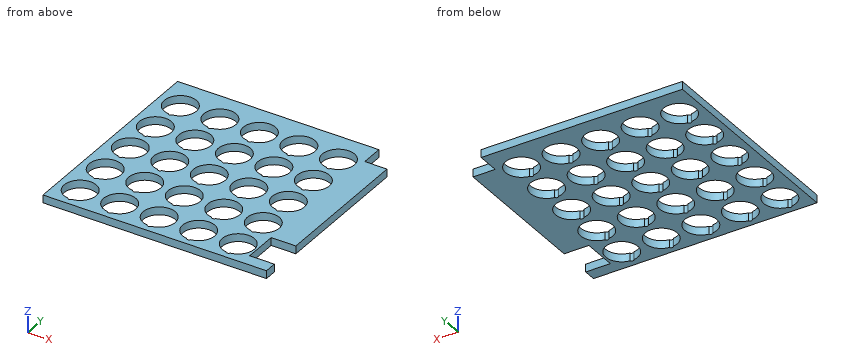
```python
from build123d import *

# Parameters (mm, degrees)
SKETCH2_W           = 180.975
SKETCH2_H           = 161.925
BOSS_EXTRUDE1_DEPTH = 6.35
SKETCH6_W           = 180.975
SKETCH6_H           = 10
BOSS_EXTRUDE2_DEPTH = 6.35
SKETCH3_R           = 13
CUT_EXTRUDE1_DEPTH  = 243.923812645
SKETCH4_R           = 1.75
CUT_EXTRUDE9_DEPTH  = 243.923812645
SKETCH7_W           = 20
SKETCH7_H           = 27.5
SKETCH7_W_2         = 18
SKETCH7_H_2         = 18
CUT_EXTRUDE10_DEPTH = 243.923812645


with BuildPart() as part:
    # Sketch2 → Boss-Extrude1 (new body)
    with BuildSketch(Plane.XY):
        with Locations((90.4875, 80.9625)):
            Rectangle(SKETCH2_W, SKETCH2_H)
    extrude(amount=BOSS_EXTRUDE1_DEPTH)

    # Sketch6 → Boss-Extrude2 (add)
    with BuildSketch(Plane.XY.offset(6.35)):
        with Locations((90.4875, -5)):
            Rectangle(SKETCH6_W, SKETCH6_H)
    extrude(amount=-BOSS_EXTRUDE2_DEPTH)

    # Sketch3 → Cut-Extrude1 (cut, through all)
    with BuildSketch(Plane.XY.offset(6.35)):
        with Locations((18.25, 8.675)):
            Circle(SKETCH3_R)
        with Locations((50.25, 8.675)):
            Circle(SKETCH3_R)
        with Locations((82.25, 8.675)):
            Circle(SKETCH3_R)
        with Locations((114.25, 8.675)):
            Circle(SKETCH3_R)
        with Locations((146.25, 8.675)):
            Circle(SKETCH3_R)
        with Locations((50.25, 40.675)):
            Circle(SKETCH3_R)
        with Locations((82.25, 40.675)):
            Circle(SKETCH3_R)
        with Locations((114.25, 40.675)):
            Circle(SKETCH3_R)
        with Locations((146.25, 40.675)):
            Circle(SKETCH3_R)
        with Locations((50.25, 72.675)):
            Circle(SKETCH3_R)
        with Locations((82.25, 72.675)):
            Circle(SKETCH3_R)
        with Locations((114.25, 72.675)):
            Circle(SKETCH3_R)
        with Locations((146.25, 72.675)):
            Circle(SKETCH3_R)
        with Locations((50.25, 104.675)):
            Circle(SKETCH3_R)
        with Locations((82.25, 104.675)):
            Circle(SKETCH3_R)
        with Locations((114.25, 104.675)):
            Circle(SKETCH3_R)
        with Locations((146.25, 104.675)):
            Circle(SKETCH3_R)
        with Locations((50.25, 136.675)):
            Circle(SKETCH3_R)
        with Locations((82.25, 136.675)):
            Circle(SKETCH3_R)
        with Locations((114.25, 136.675)):
            Circle(SKETCH3_R)
        with Locations((146.25, 136.675)):
            Circle(SKETCH3_R)
        with Locations((18.25, 40.675)):
            Circle(SKETCH3_R)
        with Locations((18.25, 72.675)):
            Circle(SKETCH3_R)
        with Locations((18.25, 104.675)):
            Circle(SKETCH3_R)
        with Locations((18.25, 136.675)):
            Circle(SKETCH3_R)
    extrude(amount=-CUT_EXTRUDE1_DEPTH, mode=Mode.SUBTRACT)

    # Sketch4 → Cut-Extrude9 (cut, through all)
    with BuildSketch(Plane.XY.offset(6.35)):
        with Locations((18.25, -3.575)):
            Circle(SKETCH4_R)
        with Locations((50.25, -3.575)):
            Circle(SKETCH4_R)
        with Locations((82.25, -3.575)):
            Circle(SKETCH4_R)
        with Locations((114.25, -3.575)):
            Circle(SKETCH4_R)
        with Locations((146.25, -3.575)):
            Circle(SKETCH4_R)
        with Locations((50.25, 28.425)):
            Circle(SKETCH4_R)
        with Locations((82.25, 28.425)):
            Circle(SKETCH4_R)
        with Locations((114.25, 28.425)):
            Circle(SKETCH4_R)
        with Locations((146.25, 28.425)):
            Circle(SKETCH4_R)
        with Locations((50.25, 60.425)):
            Circle(SKETCH4_R)
        with Locations((82.25, 60.425)):
            Circle(SKETCH4_R)
        with Locations((114.25, 60.425)):
            Circle(SKETCH4_R)
        with Locations((146.25, 60.425)):
            Circle(SKETCH4_R)
        with Locations((50.25, 92.425)):
            Circle(SKETCH4_R)
        with Locations((82.25, 92.425)):
            Circle(SKETCH4_R)
        with Locations((114.25, 92.425)):
            Circle(SKETCH4_R)
        with Locations((146.25, 92.425)):
            Circle(SKETCH4_R)
        with Locations((50.25, 124.425)):
            Circle(SKETCH4_R)
        with Locations((82.25, 124.425)):
            Circle(SKETCH4_R)
        with Locations((114.25, 124.425)):
            Circle(SKETCH4_R)
        with Locations((146.25, 124.425)):
            Circle(SKETCH4_R)
        with Locations((18.25, 28.425)):
            Circle(SKETCH4_R)
        with Locations((18.25, 60.425)):
            Circle(SKETCH4_R)
        with Locations((18.25, 92.425)):
            Circle(SKETCH4_R)
        with Locations((18.25, 124.425)):
            Circle(SKETCH4_R)
    extrude(amount=-CUT_EXTRUDE9_DEPTH, mode=Mode.SUBTRACT)

    # Sketch7 → Cut-Extrude10 (cut, through all)
    with BuildSketch(Plane.XY.offset(6.35)):
        with Locations((170.975, 13.75)):
            Rectangle(SKETCH7_W, SKETCH7_H)
        with Locations((171.975, 152.925)):
            Rectangle(SKETCH7_W_2, SKETCH7_H_2)
    extrude(amount=-CUT_EXTRUDE10_DEPTH, mode=Mode.SUBTRACT)


solid = part.part
```
Could you check a few things on this model? Use its own coordinates, in mm. Round coordinates to 2 decimals unless told otherwise and drop trailing zeros. Loops run counter-clockwise (first coordinate to the right, second up) from the corner with the lowest first, then second, coordinate; pieces in that order, holes last. Notation, with made-up numbers: (75.25, 36) -> (125.25, 36) arc R18 ccw to (125.25, 55) -> close; hole circle Ø6 at (86.25, 3). An arc over 180 degrees is marked (long way). Put each result on its own line as item: value.
Q1. For pin 1 Ø15.5 at (x, y) = (146.25, 8.675) entering from +Z; pin 2 Ø1.5 at (x, y) = (162.5, 36) entering from -Z; pin 3 Ø2 at (y, z) = (21.5, 3) entering from +X (3 decimals), each with a flat end and sliding along its axis, tell me the tip position at first contact or that it passes through.
Checks:
pin 1: through
pin 2: z = 0
pin 3: x = 160.975
Q2. I want a section at C-C on z = 5.25. Give the number of separate pieces and of enclosed holes in the cut face, and give its area (3 significant figures).
Checks:
separate pieces: 1
enclosed holes: 25
area: 16,900 mm2
Q3. I want a section at A-A on y = 17. Write out the boundary of the cut face in (x, z) (3 decimals), and give its area (3 significant figures).
Checks:
outline: (0, 0) -> (8.265, 0) -> (8.265, 6.35) -> (0, 6.35) -> close; (28.235, 0) -> (40.265, 0) -> (40.265, 6.35) -> (28.235, 6.35) -> close; (60.235, 0) -> (72.265, 0) -> (72.265, 6.35) -> (60.235, 6.35) -> close; (92.235, 0) -> (104.265, 0) -> (104.265, 6.35) -> (92.235, 6.35) -> close; (124.235, 0) -> (136.265, 0) -> (136.265, 6.35) -> (124.235, 6.35) -> close; (156.235, 0) -> (160.975, 0) -> (160.975, 6.35) -> (156.235, 6.35) -> close
area: 388 mm2
Q4. Please list where these lines run through material, in increasing order: line 1 (X direction, y = 136, z = 1) (3 decimals); line 2 (Y direction, x = 146.25, z = 5.25) (3 decimals); line 3 (X direction, y = 42.5, z = 3) (3 decimals). Write a range as from..to.
Checks:
line 1: 0..5.268, 31.232..37.268, 63.232..69.268, 95.232..101.268, 127.232..133.268, 159.232..180.975
line 2: -10..-5.325, 21.675..26.675, 53.675..58.675, 85.675..90.675, 117.675..122.675, 149.675..161.925
line 3: 0..5.379, 31.121..37.379, 63.121..69.379, 95.121..101.379, 127.121..133.379, 159.121..180.975
Q5. I want a section at B-B on x = 121. Write out the boundary of the cut face in (y, z) (3 decimals).
Checks:
outline: (-10, 0) -> (-2.435, 0) -> (-2.435, 6.35) -> (-10, 6.35) -> close; (19.785, 0) -> (29.565, 0) -> (29.565, 6.35) -> (19.785, 6.35) -> close; (51.785, 0) -> (61.565, 0) -> (61.565, 6.35) -> (51.785, 6.35) -> close; (83.785, 0) -> (93.565, 0) -> (93.565, 6.35) -> (83.785, 6.35) -> close; (115.785, 0) -> (125.565, 0) -> (125.565, 6.35) -> (115.785, 6.35) -> close; (147.785, 0) -> (161.925, 0) -> (161.925, 6.35) -> (147.785, 6.35) -> close
